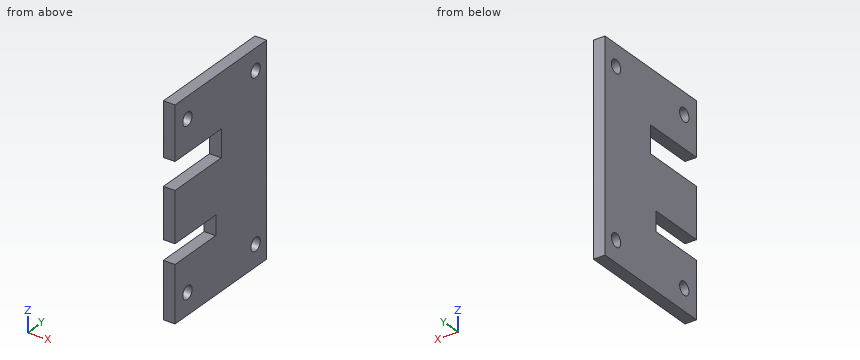
```python
from build123d import *

# Parameters (mm, degrees)
SKETCH1_W           = 53
SKETCH1_H           = 33.3
COVER_PLATE_DEPTH   = 3
SKETCH2_W           = 7
SKETCH2_H           = 17.8
SKETCH2_W_2         = 5
SKETCH2_H_2         = 15.8
CABLE_NOTCHES_DEPTH = 5
SKETCH3_R           = 1.7
SCREW_HOLES_DEPTH   = 5


with BuildPart() as part:
    # Sketch1 → Cover Plate (new body)
    with BuildSketch(Plane(origin=(72.4, 0, 0), x_dir=(0, 0, -1), z_dir=(1, 0, 0))):
        with Locations((-73, -10.15)):
            Rectangle(SKETCH1_W, SKETCH1_H)
    extrude(amount=COVER_PLATE_DEPTH)

    # Sketch2 → Cable Notches (cut)
    with BuildSketch(Plane(origin=(71.4, 0, 0), x_dir=(0, 0, -1), z_dir=(1, 0, 0))):
        with Locations((-82.3, -18.9)):
            Rectangle(SKETCH2_W, SKETCH2_H)
        with Locations((-63.4, -19.9)):
            Rectangle(SKETCH2_W_2, SKETCH2_H_2)
    extrude(amount=CABLE_NOTCHES_DEPTH, mode=Mode.SUBTRACT)

    # Sketch3 → Screw Holes (cut)
    with BuildSketch(Plane(origin=(71.4, 0, 0), x_dir=(0, 0, -1), z_dir=(1, 0, 0))):
        with Locations((-94, -22.3)):
            Circle(SKETCH3_R)
        with Locations((-94, 2.5)):
            Circle(SKETCH3_R)
        with Locations((-52, -22.3)):
            Circle(SKETCH3_R)
        with Locations((-52, 2.5)):
            Circle(SKETCH3_R)
    extrude(amount=SCREW_HOLES_DEPTH, mode=Mode.SUBTRACT)


solid = part.part
```
Could you check a few things on this model? Use its own coordinates, in mm. Coordinates: 2 decimals unless noted, no trailing zeros. Loops run counter-clockwise (first coordinate to the right, second up) from the corner with the lowest first, then second, coordinate; pieces in that order, holes last.
1) Imagine slicing it at B-B (z = 52). List the corners of the cut face in (x, y) for me, and give its area (3 significant figures).
Reported:
outline: (72.4, -26.8) - (75.4, -26.8) - (75.4, -24) - (72.4, -24) - close; (72.4, -20.6) - (75.4, -20.6) - (75.4, 0.8) - (72.4, 0.8) - close; (72.4, 4.2) - (75.4, 4.2) - (75.4, 6.5) - (72.4, 6.5) - close
area: 79.5 mm2
2) Imagine slicing it at C-C (y = 2.5). List the corners of the cut face in (x, z) for me, and give its area (3 significant figures).
Reported:
outline: (72.4, 46.5) - (75.4, 46.5) - (75.4, 50.3) - (72.4, 50.3) - close; (72.4, 53.7) - (75.4, 53.7) - (75.4, 92.3) - (72.4, 92.3) - close; (72.4, 95.7) - (75.4, 95.7) - (75.4, 99.5) - (72.4, 99.5) - close
area: 139 mm2
3) Please list where these lines run through material, in increasing order: line 1 along Z through (x, y) = (74.6, 2.5); line 2 along Z through (x, y) = (73.4, -22.3); line 3 along Y through (x, z) = (74.45, 52).
Reported:
line 1: z = 46.5 to 50.3, 53.7 to 92.3, 95.7 to 99.5
line 2: z = 46.5 to 50.3, 53.7 to 60.9, 65.9 to 78.8, 85.8 to 92.3, 95.7 to 99.5
line 3: y = -26.8 to -24, -20.6 to 0.8, 4.2 to 6.5
4) Imagine slicing it at D-D (x = 73.45). List the corners of the cut face in (y, z) for me, and give its area (3 significant figures).
Reported:
outline: (-26.8, 46.5) - (6.5, 46.5) - (6.5, 99.5) - (-26.8, 99.5) - (-26.8, 85.8) - (-10, 85.8) - (-10, 78.8) - (-26.8, 78.8) - (-26.8, 65.9) - (-12, 65.9) - (-12, 60.9) - (-26.8, 60.9) - close; hole circle Ø3.4 at (-22.3, 52); hole circle Ø3.4 at (-22.3, 94); hole circle Ø3.4 at (2.5, 52); hole circle Ø3.4 at (2.5, 94)
area: 1,540 mm2
5) Imagine slicing it at A-A (y = -22.3). List the corners of the cut face in (x, z) for me, and give its area (3 significant figures).
Reported:
outline: (72.4, 46.5) - (75.4, 46.5) - (75.4, 50.3) - (72.4, 50.3) - close; (72.4, 53.7) - (75.4, 53.7) - (75.4, 60.9) - (72.4, 60.9) - close; (72.4, 65.9) - (75.4, 65.9) - (75.4, 78.8) - (72.4, 78.8) - close; (72.4, 85.8) - (75.4, 85.8) - (75.4, 92.3) - (72.4, 92.3) - close; (72.4, 95.7) - (75.4, 95.7) - (75.4, 99.5) - (72.4, 99.5) - close
area: 103 mm2
6) Will this pin go through, and if not, where does the flat tip stop? pin 1 Ø2.5 at (y, z) = (-22.3, 52) entering from +X.
Reported:
pin 1: passes through
